Source: CAD feature listing. Evaluate the final solid. Frame: model axes, mm. Face numbers are marked on the shaded views. Round coordinates to 2 decimals unless told otherwise and drop trailing zeros. Write each loop counter-clockwise with the first axis right and the second up, starting at its lowest first coordinate (ties: lowest second). Pieces come first, ordered by that corner, then holes. Notation, with made-up numbers: (21.5, 68.5) -> (76.5, 68.5) arc R21 cw to (76.5, 93.5) -> close; hole circle Ø3 at (3.25, 55.25). An arc over 180 degrees is marked (long way). Return JSON: item names as keys, results as strings. Group by question number.
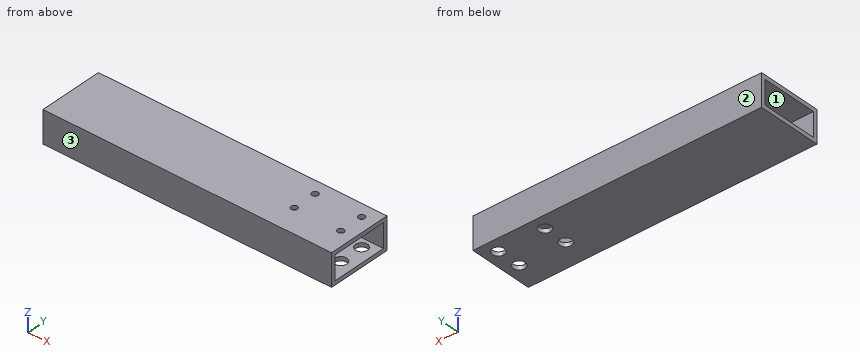
Autodesk Inventor part; units mm, degrees
ref_plane "YZ Plane" through (0, 0, 0) normal (1, 0, 0) x (0, 1, 0)
ref_plane "XZ Plane" through (0, 0, 0) normal (0, 1, 0) x (-1, 0, 0)
ref_plane "XY Plane" through (0, 0, 0) normal (0, 0, 1) x (1, 0, 0)
sketch "Sketch1" plane through (0, 0, 0) normal (1, 0, 0) x (0, 1, 0)
  line L0 (0, 0) -> (50.8, 0)
  line L1 (50.8, 0) -> (50.8, -25.4)
  line L2 (50.8, -25.4) -> (0, -25.4)
  line L3 (0, -25.4) -> (0, 0)
  line L4 (47.625, -22.225) -> (47.625, -3.175)
  line L5 (47.625, -3.175) -> (3.175, -3.175)
  line L6 (3.175, -3.175) -> (3.175, -22.225)
  line L7 (3.175, -22.225) -> (47.625, -22.225)
  dimension "d0" = 50.8
  dimension "d1" = 25.4
  dimension "d2" = 3.175
extrude "Extrusion1" add sketch "Sketch1" along normal blind 685.8
sketch "Sketch2" plane through (0, 50.8, 0) normal (0, 1, 0) x (1, 0, 0)
  line L0 (0, 0) -> (0, 25.4)
  line L1 (0, 0) -> (685.8, 0)
  line L2 (685.8, 25.4) -> (685.8, 0)
  line L3 (0, 25.4) -> (685.8, 25.4)
  line L4 (0, 0) -> (685.8, 0)
  line L5 (228.6, 0) -> (685.8, 0)
  line L6 (685.8, 0) -> (685.8, 25.4)
  line L7 (685.8, 25.4) -> (228.6, 25.4)
  line L8 (228.6, 25.4) -> (228.6, 0)
extrude "Extrusion2" cut sketch "Sketch2" against normal blind 685.8 contours L8 L3 L2 L1
hole "Hole1" at (217.805, 40.005, 0) direction (0, 0, -1) diameter 5.08 depth 12.7 tip angle 118
hole "Hole2" at (217.805, 20.955, 0) direction (0, 0, -1) diameter 5.08 depth 12.7 tip angle 118
pattern_linear "Rectangular Pattern1" count 2 spacing 36.83 along (-1, 0, 0) of "Hole1"
pattern_linear "Rectangular Pattern2" count 2 spacing 36.83 along (-1, 0, 0) of "Hole2"
hole "Hole3" at (217.805, 40.005, -25.4) direction (0, 0, 1) diameter 9.525 depth 12.7 tip angle 118
pattern_linear "Rectangular Pattern4" count 2 spacing 36.83 along (-1, 0, 0) of "Hole3"
hole "Hole4" at (217.805, 20.955, -25.4) direction (0, 0, 1) diameter 9.525 depth 12.7 tip angle 118
pattern_linear "Rectangular Pattern5" count 2 spacing 36.83 along (-1, 0, 0) of "Hole4"
properties part number "Modified Front Frame 27 in"
Item 1: Cut plane D-D on y = 40.5. Output: boundary loops of the cut face in (x, z) (3 decimals), and give its area (3 significant figures).
Item 2: First-contact query: pin 1 Ø5.5 at (x, y) = (217.805, 20.955) entering from +Z; pin 2 Ø8.5 at (x, y) = (180.975, 20.955) entering from -Z (3 decimals). Flat tips, straight axial feed; report the tip coordinate or a pass-through.
Item 3: Cut plane A-A on y = 5.5. Output: boundary loops of the cut face in (x, z) (3 decimals), and give its area (3 significant figures).
Item 4: Cut plane B-B on z = -8. Output: boundary loops of the cut face in (x, y) (3 decimals).
Item 5: Material intervals for probe 1 along Z at (x, y) = (207, 15) (3 decimals); probe 2 along Y at (x, z) = (76, -16.5) (3 decimals), sorted ascending.
Item 6: Pull-direction query (Y, two-part tool) for the marked faces 1, 2 and 3; classes: +Y half, -Y half, draft (parallel to the pull), parting line (faces both ways), or undercut.
Item 7: Cut plane C-C on x = 161. Output: boundary loops of the cut face in (y, z) (3 decimals), and give its area (3 significant figures).
Here are the results:
{
 "1": {"outline": "(0, -25.4) -> (176.238, -25.4) -> (176.238, -22.225) -> (0, -22.225) -> close; (0, -3.175) -> (178.484, -3.175) -> (178.484, 0) -> (0, 0) -> close; (183.466, -3.175) -> (215.314, -3.175) -> (215.314, 0) -> (183.466, 0) -> close; (185.712, -25.4) -> (213.068, -25.4) -> (213.068, -22.225) -> (185.712, -22.225) -> close; (220.296, -3.175) -> (228.6, -3.175) -> (228.6, 0) -> (220.296, 0) -> close; (222.542, -25.4) -> (228.6, -25.4) -> (228.6, -22.225) -> (222.542, -22.225) -> close", "area": "1,360 mm^2"},
 "2": {"pin 1": "stops at z = 0", "pin 2": "stops at z = -3.175"},
 "3": {"outline": "(0, -25.4) -> (228.6, -25.4) -> (228.6, -22.225) -> (0, -22.225) -> close; (0, -3.175) -> (228.6, -3.175) -> (228.6, 0) -> (0, 0) -> close", "area": "1,450 mm^2"},
 "4": {"outline": "(0, 0) -> (228.6, 0) -> (228.6, 3.175) -> (0, 3.175) -> close; (0, 47.625) -> (228.6, 47.625) -> (228.6, 50.8) -> (0, 50.8) -> close"},
 "5": {"probe 1": "z = -25.4 to -22.225, -3.175 to 0", "probe 2": "y = 0 to 3.175, 47.625 to 50.8"},
 "6": {"face 1": "undercut", "face 2": "+Y half", "face 3": "-Y half"},
 "7": {"outline": "(0, -25.4) -> (50.8, -25.4) -> (50.8, 0) -> (0, 0) -> close; hole (3.175, -22.225) -> (47.625, -22.225) -> (47.625, -3.175) -> (3.175, -3.175) -> close", "area": "444 mm^2"}
}
